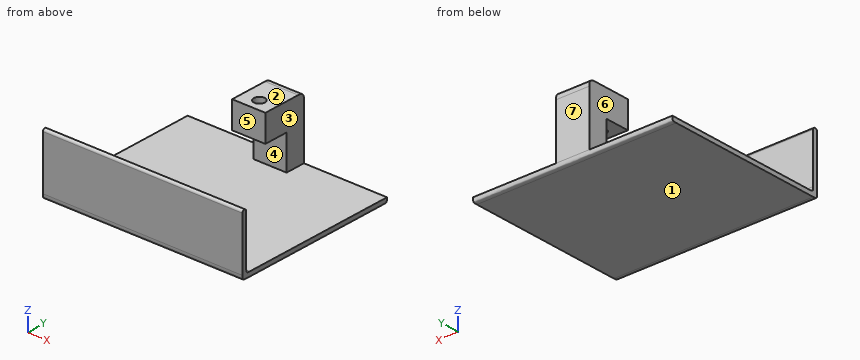
```python
from build123d import *

# Parameters (mm, degrees)
SKETCH1_W           = 75
SKETCH1_H           = 60
BOSS_EXTRUDE2_DEPTH = 100
SKETCH2_W           = 75
SKETCH2_H           = 45
BOSS_EXTRUDE3_DEPTH = 77.5
BOSS_EXTRUDE4_DEPTH = 10
SKETCH4_W           = 450
SKETCH4_H           = 10
BOSS_EXTRUDE5_DEPTH = 125
SKETCH5_R           = 12.5
CUT_EXTRUDE1_DEPTH  = 125
FILLET3_SIZE        = 10
FILLET4_RADIUS      = 5
FILLET4_LENGTH      = 450
FILLET5_SIZE        = 10
FILLET6_SIZE        = 15


with BuildPart() as part:
    # Sketch1 → Boss-Extrude2 (new body)
    with BuildSketch(Plane(origin=(0, 0, 0), x_dir=(1, 0, 0), z_dir=(0, 1, 0))):
        Rectangle(SKETCH1_W, SKETCH1_H)
    extrude(amount=BOSS_EXTRUDE2_DEPTH)

    # Sketch2 → Boss-Extrude3 (add)
    with BuildSketch(Plane(origin=(0, 0, -30), x_dir=(-1, 0, 0), z_dir=(0, 0, -1))):
        with Locations((0, 77.5)):
            Rectangle(SKETCH2_W, SKETCH2_H)
    extrude(amount=BOSS_EXTRUDE3_DEPTH)

    # Sketch3 → Boss-Extrude4 (add)
    with BuildSketch(Plane(origin=(0, 0, -107.5), x_dir=(-1, 0, 0), z_dir=(0, 0, -1))):
        Polygon((0, 100), (225, 100), (225, -275), (25, -275), (-225, -275), (-225, 100), align=None)
    extrude(amount=BOSS_EXTRUDE4_DEPTH)

    # Sketch4 → Boss-Extrude5 (add)
    with BuildSketch(Plane.XY.offset(-107.5)):
        with Locations((0, -270)):
            Rectangle(SKETCH4_W, SKETCH4_H)
    extrude(amount=BOSS_EXTRUDE5_DEPTH)

    # Sketch5 → Cut-Extrude1 (cut)
    with BuildSketch(Plane.XY.offset(30)):
        with Locations((0, 27.501368098)):
            Circle(SKETCH5_R)
    extrude(amount=-CUT_EXTRUDE1_DEPTH, mode=Mode.SUBTRACT)

    # Fillet3
    # a fillet whose section is not a circle: 10 mm, written as the material it takes off along each edge
    with BuildSketch(Plane(origin=(-250, -275, -117.5), x_dir=(0, 1, 0), z_dir=(1, 0, 0))) as fillet3_piece_1:
        with BuildLine():
            Bezier((FILLET3_SIZE, 0), (0, 0), (0, FILLET3_SIZE), weights=[1, 2.333333333, 1])
            Line((0, FILLET3_SIZE), (0, 0))
            Line((0, 0), (FILLET3_SIZE, 0))
        make_face()
    extrude(amount=500, mode=Mode.SUBTRACT)
    with BuildSketch(Plane(origin=(250, 100, -117.5), x_dir=(0, 0, 1), z_dir=(-1, 0, 0))) as fillet3_piece_2:
        with BuildLine():
            Bezier((FILLET3_SIZE, 0), (0, 0), (0, -FILLET3_SIZE), weights=[1, 2.333333333, 1])
            Line((0, -FILLET3_SIZE), (0, 0))
            Line((0, 0), (FILLET3_SIZE, 0))
        make_face()
    extrude(amount=500, mode=Mode.SUBTRACT)

    # Fillet4: full round fillet: the end face becomes a half cylinder, R = half its width
    fillet4_face = Plane((0, -270, 17.5), x_dir=(1, 0, 0), z_dir=(0, 0, 1))  # on the end face: x along it, z out of the body
    fillet4_slab = fillet4_face.offset(-FILLET4_RADIUS / 2) * Box(FILLET4_LENGTH, 2 * FILLET4_RADIUS, FILLET4_RADIUS, mode=Mode.PRIVATE)  # the body's end, R deep
    fillet4_round = Plane((0, -270, 12.5), x_dir=(0, 0, 1), z_dir=(1, 0, 0)) * Cylinder(FILLET4_RADIUS, FILLET4_LENGTH, mode=Mode.PRIVATE)  # its axis R under the face
    add(fillet4_slab - fillet4_round, mode=Mode.SUBTRACT)

    # Fillet5
    # a fillet whose section is not a circle: 10 mm, written as the material it adds along each edge
    with BuildSketch(Plane(origin=(225, -265, -107.5), x_dir=(0, 1, 0), z_dir=(-1, 0, 0))) as fillet5_piece_1:
        with BuildLine():
            Bezier((FILLET5_SIZE, 0), (0, 0), (0, -FILLET5_SIZE), weights=[1, 2.333333333, 1])
            Line((0, -FILLET5_SIZE), (-FILLET5_SIZE * 0.02, -FILLET5_SIZE))
            Line((-FILLET5_SIZE * 0.02, -FILLET5_SIZE), (-FILLET5_SIZE * 0.02, FILLET5_SIZE * 0.02))
            Line((-FILLET5_SIZE * 0.02, FILLET5_SIZE * 0.02), (FILLET5_SIZE, FILLET5_SIZE * 0.02))
            Line((FILLET5_SIZE, FILLET5_SIZE * 0.02), (FILLET5_SIZE, 0))
        make_face()
    extrude(amount=450)

    # Fillet6
    # a fillet whose section is not a circle: 15 mm, written as the material it takes off along each edge
    with BuildSketch(Plane(origin=(-75, 100, 30), x_dir=(0, 0, -1), z_dir=(1, 0, 0))) as fillet6_piece_1:
        with BuildLine():
            add(Edge.make_bspline([(FILLET6_SIZE, 0), (FILLET6_SIZE * 0.831801948466, 0), (FILLET6_SIZE * 0.663603896932, 0), (FILLET6_SIZE * 0.292893218813, -FILLET6_SIZE * 0.0716919198361), (FILLET6_SIZE * 0.0716919198361, -FILLET6_SIZE * 0.292893218813), (0, -FILLET6_SIZE * 0.663603896932), (0, -FILLET6_SIZE * 0.831801948466), (0, -FILLET6_SIZE)], knots=[0, 0, 0, 0, 0, 0, 0.5, 0.5, 1, 1, 1, 1, 1, 1], degree=5))
            Line((0, -FILLET6_SIZE), (0, 0))
            Line((0, 0), (FILLET6_SIZE, 0))
        make_face()
    extrude(amount=150, mode=Mode.SUBTRACT)


solid = part.part
```
Geometry check sheet. Reference: the model listing, model coordinates, mm. Face numbers are marked on the shaded views. A direction names the side the tool comes from. Coordinates: 2 decimals unless noted, no trailing zeros. Order: outer loops, then holes, each group sorted by start corner. A loop starts at its lowest first (then second) coordinate and runs counter-clockwise, first axis right, second up. Notation, with made-up numbers: (56, -37) - (69, -37) arc R16 ccw to (69, -23) - close; hole circle Ø7 at (89.25, 55). An arc over 180 degrees is marked (long way). Answer as a JSON object with one key per item and string values. Group by question number.
Item 1: Draft check along Z on the marked faces 1, 2, 3 and 4. Enter one of: +Z half, -Z half, draft (parallel to the pull), parting line (faces both ways), or undercut.
Item 2: Sectioned sample at A-A, the plane z = -37. Record the cut outline in (x, y).
Item 3: Sectioned sample at C-C, the plane y = -119. Record the cut outline in (x, z), and give its area (3 significant figures).
Item 4: Scan lines: probe 1 along Y at (x, z) = (0, -2); probe 2 along Z at (x, y) = (-18, 38); probe 3 along Y at (x, z) = (-195, -91). Record each from-to range of solid material in increasing order.
Item 5: Tool access check on the marked faces 5, 6 and 7. Record the directions out of +Z, -Z, +X, -X, +Y, -Y that give a thin tool (end or side, any length) a straight path to the whole face; none if there is none.
Item 6: Sectioned sample at B-B, the plane y = 70.5. Record the cut outline in (x, z), and give its area (3 significant figures).
Item 7: Depth check by flat-ended pin: pin 1 Ø12 at (x, z) = (136.5, 7) entering from +Y. Enter the tip coordinate at first touch or a pass-through.
Resolved:
{
 "1": {"face 1": "-Z half", "face 2": "+Z half", "face 3": "draft", "face 4": "undercut"},
 "2": {"outline": "(-225, -275) - (225, -275) - (225, -265) - (-225, -265) - close; (-37.5, 55) - (37.5, 55) - (37.5, 100) - (-37.5, 100) - close"},
 "3": {"outline": "(-225, -117.5) - (225, -117.5) - (225, -107.5) - (-225, -107.5) - close", "area": "4,500 mm^2"},
 "4": {"probe 1": "-275 to -265, 0 to 15, 40 to 100", "probe 2": "-117.5 to -107.5, -30 to 30", "probe 3": "-275 to -265"},
 "5": {"face 5": "+Z, +X, -X", "face 6": "+Z, -X, +Y", "face 7": "+Z, -Z, +X, -X, +Y"},
 "6": {"outline": "(-225, -117.5) - (225, -117.5) - (225, -107.5) - (37.5, -107.5) - (37.5, 30) - (-37.5, 30) - (-37.5, -107.5) - (-225, -107.5) - close", "area": "14,800 mm^2"},
 "7": {"pin 1": "y = -265"}
}
